Check sheet for the modelled part. Datum: model origin and axes. Units: mm. Face numbers are marked on the shaded views. A direction names the side the tool comes from. Coordinates: 2 decimals unless noted, no trailing zeros. Loops run counter-clockwise (first coordinate to the right, second up) from the corner with the lowest first, then second, coordinate; pieces in that order, holes last. Notation, with made-up numbers: (68, -32) - (91, -32) arc R15 cw to (91, -11) - close; hole circle Ø2 at (24, 84). An arc over 180 degrees is marked (long way). Use a Markdown table: item, result. Add a question column.
1) Go/stop test with flat-tipped pins: P1, Ø2, axis at x = 34.5, z = 28, coming from the +Y side; P2, Ø2, axis at x = 19.5, z = 31, coming from the +Y side; P3, Ø9.5, axis at x = 34, y = 45.5, coming from the +Z side. Record where each tip stops, or that it passes through.
2) Sectioned sample at D-D, the plane z = 10. Enter the section's corners in (x, y), then the cut area to 3 significant figures.
3) Draft check along X on the marked faces 1, 2, 3 and 4. Enter one of: pulls with the +X half, pulls with the -X half, needs draft (parallel to the pull), parting line crosses it, or undercut.
4) Thickness scan on line 1 (Y direction, x = 52, z = 9.5); line 2 (Y direction, x = 28, z = 2); line 3 (X direction, y = 45.5, z = 38). Record the ranges inside material, lowest first.
5) Sectioned sample at A-A, the plane y = 28.5. Enter the section's corners in (x, z), then the cut area to 3 significant figures.
6) Sectioned sample at B-B, the plane x = 28.5. Enter the section's corners in (y, z), then the cut area to 3 significant figures.
7) Tool access check on the marked faces 5 and 6. Record the directions out of +Z, -Z, +X, -X, +Y, -Y that give a thin tool (end or side, any length) a straight path to the whole face; none if there is none.
8) Sectioned sample at C-C, the plane y = 53. Enter the section's corners in (x, z).
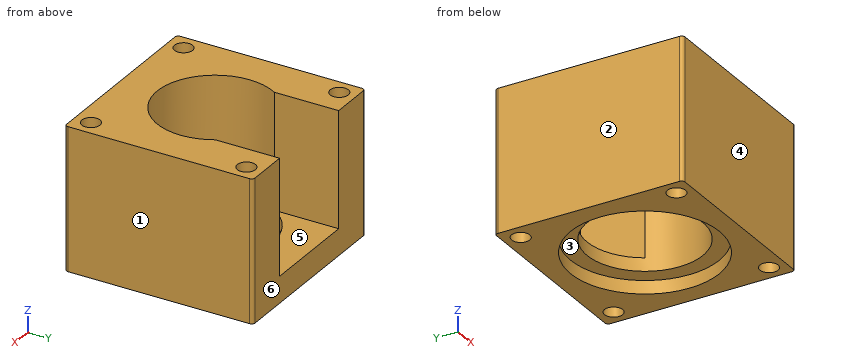
from build123d import *

# Parameters (mm, degrees)
ESQUISSE1_R             = 17.5
ESQUISSE1_R_2           = 2.75
BOSS_EXTRU_1_DEPTH      = 43
ESQUISSE2_W             = 30
ESQUISSE2_H             = 35
ENL_V_MAT_EXTRU_1_DEPTH = 30
ESQUISSE3_R             = 22.5
ENL_V_MAT_EXTRU_2_DEPTH = 4


with BuildPart() as part:
    # Esquisse1 → Boss.-Extru.1 (new body)
    with BuildSketch(Plane.XY):
        with BuildLine():
            Line((1, 0), (56, 0))
            ThreePointArc((56, 0), (56.707106781, 0.292893219), (57, 1))
            Line((57, 1), (57, 56))
            ThreePointArc((57, 56), (56.707106781, 56.707106781), (56, 57))
            Line((56, 57), (1, 57))
            ThreePointArc((1, 57), (0.292893219, 56.707106781), (0, 56))
            Line((0, 56), (0, 1))
            ThreePointArc((0, 1), (0.292893219, 0.292893219), (1, 0))
        make_face()
        with Locations((28.5, 28.5)):
            Circle(ESQUISSE1_R, mode=Mode.SUBTRACT)
        with Locations((4.926655582, 52.073344418)):
            Circle(ESQUISSE1_R_2, mode=Mode.SUBTRACT)
        with Locations((52.026632419, 52.026632419)):
            Circle(ESQUISSE1_R_2, mode=Mode.SUBTRACT)
        with Locations(Location((4.926655582, 4.926655582, 0), (0, 0, 180))):
            Circle(ESQUISSE1_R_2, mode=Mode.SUBTRACT)
        with Locations(Location((52.026632419, 4.973367581, 0), (0, 0, 180))):
            Circle(ESQUISSE1_R_2, mode=Mode.SUBTRACT)
    extrude(amount=BOSS_EXTRU_1_DEPTH)

    # Esquisse2 → Enlèv. mat.-Extru.1 (cut)
    with BuildSketch(Plane(origin=(0, 57, 0), x_dir=(1, 0, 0), z_dir=(0, 1, 0))):
        with Locations((28.5, -25.5)):
            Rectangle(ESQUISSE2_W, ESQUISSE2_H)
    extrude(amount=-ENL_V_MAT_EXTRU_1_DEPTH, mode=Mode.SUBTRACT)

    # Esquisse3 → Enlèv. mat.-Extru.2 (cut)
    with BuildSketch(Plane(origin=(0, 0, 0), x_dir=(-1, 0, 0), z_dir=(0, 0, -1))):
        with Locations((-28.5, 28.5)):
            Circle(ESQUISSE3_R)
    extrude(amount=-ENL_V_MAT_EXTRU_2_DEPTH, mode=Mode.SUBTRACT)


solid = part.part
Solved:
| question | item | result |
|---|---|---|
| 1 | P1 | stops at y = 12.46 |
| 1 | P2 | stops at y = 14.14 |
| 1 | P3 | stops at z = 8 |
| 2 | outline | (0, 1) arc R1 ccw to (1, 0) - (56, 0) arc R1 ccw to (57, 1) - (57, 56) arc R1 ccw to (56, 57) - (43.5, 57) - (43.5, 37.51) arc R17.5 cw (long way) to (13.5, 37.51) - (13.5, 57) - (1, 57) arc R1 ccw to (0, 56) - close; hole circle Ø5.5 at (4.93, 4.93); hole circle Ø5.5 at (4.93, 52.07); hole circle Ø5.5 at (52.03, 4.97); hole circle Ø5.5 at (52.03, 52.03) |
| 2 | area | 1,790 mm2 |
| 3 | face 1 | pulls with the +X half |
| 3 | face 2 | pulls with the -X half |
| 3 | face 3 | undercut |
| 3 | face 4 | needs draft |
| 4 | line 1 | y = 0 to 2.22, 7.72 to 49.28, 54.78 to 57 |
| 4 | line 2 | y = 0 to 6.01, 50.99 to 57 |
| 4 | line 3 | x = 0 to 13.5, 43.5 to 57 |
| 5 | outline | (0, 0) - (6, 0) - (6, 4) - (11, 4) - (11, 43) - (0, 43) - close; (46, 4) - (51, 4) - (51, 0) - (57, 0) - (57, 43) - (46, 43) - close |
| 5 | area | 906 mm2 |
| 6 | outline | (0, 0) - (6, 0) - (6, 4) - (11, 4) - (11, 43) - (0, 43) - close; (46, 4) - (51, 4) - (51, 0) - (57, 0) - (57, 8) - (46, 8) - close |
| 6 | area | 521 mm2 |
| 7 | face 5 | +Z, +Y |
| 7 | face 6 | +Z, -Z, +X, -X, +Y |
| 8 | outline | (0, 0) - (2.34, 0) - (2.34, 43) - (0, 43) - close; (7.52, 0) - (49.45, 0) - (49.45, 43) - (43.5, 43) - (43.5, 8) - (13.5, 8) - (13.5, 43) - (7.52, 43) - close; (54.6, 0) - (57, 0) - (57, 43) - (54.6, 43) - close |
